Autodesk Fusion 360 part; units mm, degrees
sketch "Sketch1" plane through (0, 0, 0) normal (0, 0, 1) x (1, 0, 0)
  line L0 (12.5, 13.5) -> (-12.5, 13.5)
  line L1 (-12.5, 13.5) -> (-12.5, -13.5)
  line L2 (-12.5, -13.5) -> (12.5, -13.5)
  line L3 (12.5, -13.5) -> (12.5, 13.5)
  line L4 (12.5, -13.5) -> (-12.5, 13.5) construction
  dimension "d1" = 25
  dimension "d2" = 27
extrude "Extrude1" add sketch "Sketch1" along normal blind 1
sketch "Sketch2" plane through (0, 0, 0) normal (0, 0, -1) x (1, 0, 0)
  line L0 (12.5, -13.5) -> (12.5, 13.5)
  line L1 (12.5, 13.5) -> (-12.5, 13.5)
  line L2 (-12.5, 13.5) -> (-12.5, -13.5)
  line L3 (-12.5, -13.5) -> (12.5, -13.5)
  line L4 (-5.08, 10.96) -> (5.08, 10.96)
  line L5 (5.08, 10.96) -> (5.08, 13.5)
  line L6 (5.08, 13.5) -> (-5.08, 13.5)
  line L7 (-5.08, 13.5) -> (-5.08, 10.96)
  dimension "d5" = 2.54
  dimension "d6" = 10.16
extrude "Extrude2" add sketch "Sketch2" along normal blind 2.54 contours L1 L4 L5 L6 L7
sketch "Sketch3" plane through (0, 0, 1) normal (0, 0, 1) x (-1, 0, 0)
  line L0 (-12.5, 13.5) -> (-12.5, -13.5)
  line L1 (-12.5, -13.5) -> (12.5, -13.5)
  line L2 (12.5, -13.5) -> (12.5, 13.5)
  line L3 (12.5, 13.5) -> (-12.5, 13.5)
  line L4 (12.5, 8.5) -> (-12.5, 8.5)
  line L5 (-12.5, 8.5) -> (-12.5, -8.5)
  line L6 (-12.5, -8.5) -> (12.5, -8.5)
  line L7 (12.5, -8.5) -> (12.5, 8.5)
  line L8 (0, 8.5) -> (0, 13.5) construction
  dimension "d9" = 17
  dimension "d10" = 5
extrude "Extrude3" add sketch "Sketch3" along normal blind 1.6 contours L0 L2 L4 L5 L6 L7
Source: CAD feature listing. Evaluate the final solid. Frame: model axes, mm. A direction names the side the tool comes from. Give positions to 0.01 mm unless a question says otherwise; leave off trailing zeros. Write each loop counter-clockwise with the first axis right and the second up, starting at its lowest first coordinate (ties: lowest second). Pieces come first, ordered by that corner, then holes. Notation, with made-up numbers: (-3.5, 4.5) - (44.5, 4.5) arc R21 ccw to (44.5, 33.5) - close; hole circle Ø8 at (26, 53). An arc over 180 degrees is marked (long way). Write item = value, one per line. Start each with the question number.
Q1. Cut plane C-C, the plane x = -8.75. Return loops of the section in (y, z).
Q2. Reachability of faces 1 (the flat face through (0, 8.5, 2)), 2 (the flat face through (0, -11, 1)), 3 (the flat face through (-5.08, -12, -1)), 4 (the flat face through (0, -10.96, -1)) from +Z, -Z, +X, -X, +Y, -Y: full face, straight path, thin tool, end or side. Return the list, or none.
Q3. Material intervals for probe 1 along Z at (x, y) = (8.75, -1.5); probe 2 along Z at (x, y) = (7.75, 11.5); probe 3 along X at (y, z) = (-11.75, -0.65), sorted ascending.
Q4. Cut plane A-A, the plane x = -4.75. Return loops of the section in (y, z), then the cut area to 3 significant figures.
Q5. Cut plane B-B, the plane y = 7.75. Return loops of the section in (x, z).
Q6. Pin query (flat end, axial travel): pin 1 Ø0.5 at (x, z) = (4.5, 1.5) entering from -Y; pin 2 Ø3 at (x, z) = (5.5, -1.5) entering from -Y; pin 3 Ø1.3 at (x, z) = (-1, -1.5) entering from +Y; pin 4 Ø0.5 at (x, z) = (6, 2) entering from +Y. Return the tip coordinate at first contact, or that it passes through.
Q7. Cut plane D-D, the plane z = 1.35. Return loops of the section in (x, y), then the cut area to 3 significant figures.
Computed values:
q1.outline = (-13.5, 0) - (13.5, 0) - (13.5, 1) - (8.5, 1) - (8.5, 2.6) - (-8.5, 2.6) - (-8.5, 1) - (-13.5, 1) - close
q2.face_1 = +Z, +X, -X, +Y
q2.face_2 = +Z, +X, -X, -Y
q2.face_3 = -Z, -X, +Y, -Y
q2.face_4 = -Z, +X, -X, +Y
q3.probe_1 = 0 to 2.6
q3.probe_2 = 0 to 1
q3.probe_3 = -5.08 to 5.08
q4.outline = (-13.5, -2.54) - (-10.96, -2.54) - (-10.96, 0) - (13.5, 0) - (13.5, 1) - (8.5, 1) - (8.5, 2.6) - (-8.5, 2.6) - (-8.5, 1) - (-13.5, 1) - close
q4.area = 60.7 mm²
q5.outline = (-12.5, 0) - (12.5, 0) - (12.5, 2.6) - (-12.5, 2.6) - close
q6.pin_1 = -8.5
q6.pin_2 = -13.5
q6.pin_3 = -10.96
q6.pin_4 = 8.5
q7.outline = (-12.5, -8.5) - (12.5, -8.5) - (12.5, 8.5) - (-12.5, 8.5) - close
q7.area = 425 mm²
